For this review, take the finished solid that the model builds, in its own axes (mm). Face numbers are marked on the shaded views. A direction names the side the tool comes from. Coordinates: 2 decimals unless noted, no trailing zeros. Write each loop counter-clockwise with the first axis right and the second up, starting at its lowest first coordinate (ties: lowest second). Pieces come first, ordered by that corner, then holes. Notation, with made-up numbers: M 16,16.5 L 46,16.5 A17 cw 46,46.5 Z; hole C 6.5,9 d10. An arc over 180 degrees is marked long. Return JSON: item names as keys, results as strings.
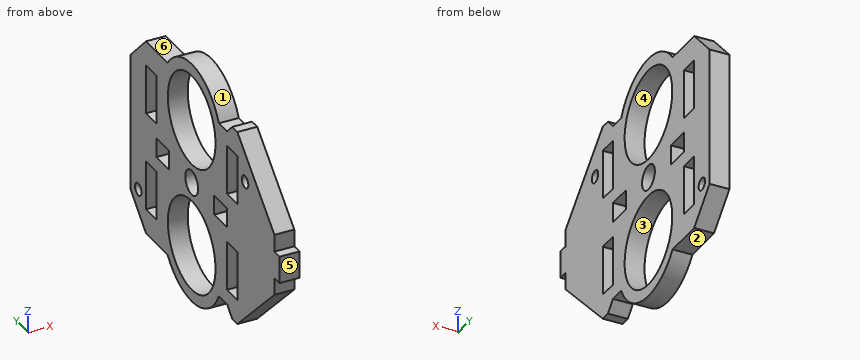
```python
from build123d import *

# Parameters (mm, degrees)
SKETCH1_R           = 2.5
SKETCH1_R_2         = 18.5
SKETCH1_R_3         = 5
BOSS_EXTRUDE1_DEPTH = 8
CUT_EXTRUDE1_REACH  = 86.69
SKETCH2_W           = 20
SKETCH2_H           = 8
SKETCH2_W_2         = 8
SKETCH2_H_2         = 10
SKETCH2_W_3         = 7
SKETCH2_H_3         = 4


with BuildPart() as part:
    # Sketch1 → Boss-Extrude1 (new body)
    with BuildSketch(Plane(origin=(0, 0, 0), x_dir=(0, 0, -1), z_dir=(1, 0, 0))):
        with BuildLine():
            Line((-12.5, -64.29), (-40, -35.5))
            Line((-40, -35.5), (-40, -31.5))
            Line((-40, -31.5), (-36, -27.5))
            Line((-36, -27.5), (-36, -21.143055078))
            ThreePointArc((-36, -21.143055078), (-49.329627244, -2.32877567), (-40, 18.757099403))
            Line((-40, 18.757099403), (-40, 35.5))
            Line((-40, 35.5), (-28, 47.5))
            Line((-28, 47.5), (28, 47.5))
            Line((28, 47.5), (40, 35.5))
            Line((40, 35.5), (40, 18.757099403))
            ThreePointArc((40, 18.757099403), (49.329627244, -2.32877567), (36, -21.143055078))
            Line((36, -21.143055078), (36, -27.5))
            Line((36, -27.5), (40, -31.5))
            Line((40, -31.5), (40, -35.5))
            Line((40, -35.5), (12.5, -64.29))
            Line((12.5, -64.29), (12.5, -68.29))
            Line((12.5, -68.29), (-12.5, -68.29))
            Line((-12.5, -68.29), (-12.5, -64.29))
        make_face()
        with Locations((-22.373880505, -41.5)):
            Circle(SKETCH1_R, mode=Mode.SUBTRACT)
        with Locations((24.891578032, 41.5)):
            Circle(SKETCH1_R, mode=Mode.SUBTRACT)
        with Locations((-26.1, 0)):
            Circle(SKETCH1_R_2, mode=Mode.SUBTRACT)
        with Locations(Location((26.1, 0, 0), (0, 0, 180))):
            Circle(SKETCH1_R_2, mode=Mode.SUBTRACT)
        Circle(SKETCH1_R_3, mode=Mode.SUBTRACT)
    extrude(amount=BOSS_EXTRUDE1_DEPTH)

    # Sketch2 → Cut-Extrude1 (cut, up to next)
    with BuildSketch(Plane.ZY, mode=Mode.PRIVATE) as cut_extrude1_sk1:
        with Locations((20, -31.5)):
            Rectangle(SKETCH2_W, SKETCH2_H)
    cut_extrude1_tool1 = extrude(cut_extrude1_sk1.sketch, amount=-CUT_EXTRUDE1_REACH, mode=Mode.PRIVATE) & part.part
    # Sketch2 → Cut-Extrude1 (cut, up to next)
    with BuildSketch(Plane.ZY, mode=Mode.PRIVATE) as cut_extrude1_sk2:
        with Locations((-20, -31.5)):
            Rectangle(SKETCH2_W, SKETCH2_H)
    cut_extrude1_tool2 = extrude(cut_extrude1_sk2.sketch, amount=-CUT_EXTRUDE1_REACH, mode=Mode.PRIVATE) & part.part
    # Sketch2 → Cut-Extrude1 (cut, up to next)
    with BuildSketch(Plane.ZY, mode=Mode.PRIVATE) as cut_extrude1_sk3:
        with Locations((20, 31.5)):
            Rectangle(SKETCH2_W, SKETCH2_H)
    cut_extrude1_tool3 = extrude(cut_extrude1_sk3.sketch, amount=-CUT_EXTRUDE1_REACH, mode=Mode.PRIVATE) & part.part
    # Sketch2 → Cut-Extrude1 (cut, up to next)
    with BuildSketch(Plane.ZY, mode=Mode.PRIVATE) as cut_extrude1_sk4:
        with Locations((-20, 31.5)):
            Rectangle(SKETCH2_W, SKETCH2_H)
    cut_extrude1_tool4 = extrude(cut_extrude1_sk4.sketch, amount=-CUT_EXTRUDE1_REACH, mode=Mode.PRIVATE) & part.part
    # Sketch2 → Cut-Extrude1 (cut, up to next)
    with BuildSketch(Plane.ZY, mode=Mode.PRIVATE) as cut_extrude1_sk5:
        with Locations((0, 22.5)):
            Rectangle(SKETCH2_W_2, SKETCH2_H_2)
    cut_extrude1_tool5 = extrude(cut_extrude1_sk5.sketch, amount=-CUT_EXTRUDE1_REACH, mode=Mode.PRIVATE) & part.part
    # Sketch2 → Cut-Extrude1 (cut, up to next)
    with BuildSketch(Plane.ZY, mode=Mode.PRIVATE) as cut_extrude1_sk6:
        with Locations((0, -22.5)):
            Rectangle(SKETCH2_W_2, SKETCH2_H_2)
    cut_extrude1_tool6 = extrude(cut_extrude1_sk6.sketch, amount=-CUT_EXTRUDE1_REACH, mode=Mode.PRIVATE) & part.part
    # Sketch2 → Cut-Extrude1 (cut, up to next)
    with BuildSketch(Plane.ZY, mode=Mode.PRIVATE) as cut_extrude1_sk7:
        with Locations((9, -66.29)):
            Rectangle(SKETCH2_W_3, SKETCH2_H_3)
    cut_extrude1_tool7 = extrude(cut_extrude1_sk7.sketch, amount=-CUT_EXTRUDE1_REACH, mode=Mode.PRIVATE) & part.part
    # Sketch2 → Cut-Extrude1 (cut, up to next)
    with BuildSketch(Plane.ZY, mode=Mode.PRIVATE) as cut_extrude1_sk8:
        with Locations((-9, -66.29)):
            Rectangle(SKETCH2_W_3, SKETCH2_H_3)
    cut_extrude1_tool8 = extrude(cut_extrude1_sk8.sketch, amount=-CUT_EXTRUDE1_REACH, mode=Mode.PRIVATE) & part.part
    add(cut_extrude1_tool1.solids().sort_by_distance((0, -31.5, 20))[0], mode=Mode.SUBTRACT)
    add(cut_extrude1_tool2.solids().sort_by_distance((0, -31.5, -20))[0], mode=Mode.SUBTRACT)
    add(cut_extrude1_tool3.solids().sort_by_distance((0, 31.5, 20))[0], mode=Mode.SUBTRACT)
    add(cut_extrude1_tool4.solids().sort_by_distance((0, 31.5, -20))[0], mode=Mode.SUBTRACT)
    add(cut_extrude1_tool5.solids().sort_by_distance((0, 22.5, 0))[0], mode=Mode.SUBTRACT)
    add(cut_extrude1_tool6.solids().sort_by_distance((0, -22.5, 0))[0], mode=Mode.SUBTRACT)
    add(cut_extrude1_tool7.solids().sort_by_distance((0, -66.29, 9))[0], mode=Mode.SUBTRACT)
    add(cut_extrude1_tool8.solids().sort_by_distance((0, -66.29, -9))[0], mode=Mode.SUBTRACT)


solid = part.part
```
1. We need section B-B (z = 0). State the section outline as (x, y) points.
Checks:
{"outline": "M 0,-68.29 L 8,-68.29 L 8,-27.5 L 0,-27.5 Z; M 0,-17.5 L 8,-17.5 L 8,-5 L 0,-5 Z; M 0,5 L 8,5 L 8,17.5 L 0,17.5 Z; M 0,27.5 L 8,27.5 L 8,47.5 L 0,47.5 Z"}
2. For the marked faces 5 and 6, list the 3-axis set-ups (+Z, -Z, +X, -X, +Y, -Y) from which the entire face can be reached by the end or side of a thin tool; tool diameter is ignored.
Checks:
{"face 5": "+Z, -Z, +X, -X, -Y", "face 6": "+Z, +X, -X, +Y"}
3. Draft analysis for pull direction Z (two halves, no side actions). For the marked faces 1, 2, 3 and 4, state which applies: +Z half, -Z half, draft (parallel to the pull), parting line (faces both ways), or undercut.
Checks:
{"face 1": "+Z half", "face 2": "-Z half", "face 3": "undercut", "face 4": "undercut"}
4. We need section A-A (y = 0). State the section outline as (x, z) points.
Checks:
{"outline": "M 0,-49.45 L 8,-49.45 L 8,-44.6 L 0,-44.6 Z; M 0,-7.6 L 8,-7.6 L 8,-5 L 0,-5 Z; M 0,5 L 8,5 L 8,7.6 L 0,7.6 Z; M 0,44.6 L 8,44.6 L 8,49.45 L 0,49.45 Z"}
5. Clearance check with flat-ended pins moving along their axes: pin 1 Ø4 at (x, y) = (3, 30.5) entering from +Z; pin 2 Ø1 at (x, z) = (3, -32) entering from +Y; pin 3 Ø4 at (x, z) = (5, -18) entering from -Y. State where each tip first meets the part, or that it passes through.
Checks:
{"pin 1": "z = 40", "pin 2": "y = 44", "pin 3": "y = -60.63"}
6. We need section D-D (z = 23). State the section outline as (x, y) points, plus the area to 3 significant figures.
Checks:
{"outline": "M 0,-53.3 L 8,-53.3 L 8,-43.92 L 0,-43.92 Z; M 0,-39.08 L 8,-39.08 L 8,-35.5 L 0,-35.5 Z; M 0,-27.5 L 8,-27.5 L 8,-18.24 L 0,-18.24 Z; M 0,18.24 L 8,18.24 L 8,27.5 L 0,27.5 Z; M 0,35.5 L 8,35.5 L 8,47.5 L 0,47.5 Z", "area": "348 mm2"}
7. We need section C-C (y = 41.5). State the section outline as (x, z) points.
Checks:
{"outline": "M 0,-34 L 8,-34 L 8,-27.39 L 0,-27.39 Z; M 0,-22.39 L 8,-22.39 L 8,34 L 0,34 Z"}
8. Wall thickness on L1, parallel to Z at x = 4.5, y = 31.5; L2, parallel to Y at x = 3, z = 0; L3, parallel to Y at x = 4.75, z = -14: over which ranges is each line inside the solid? List them lowest first. Write a range as from..to.
Checks:
{"L1": "-40..-30, -10..10, 30..40", "L2": "-68.29..-27.5, -17.5..-5, 5..17.5, 27.5..47.5", "L3": "-62.72..-35.5, -27.5..-13.99, 13.99..27.5, 35.5..47.5"}
